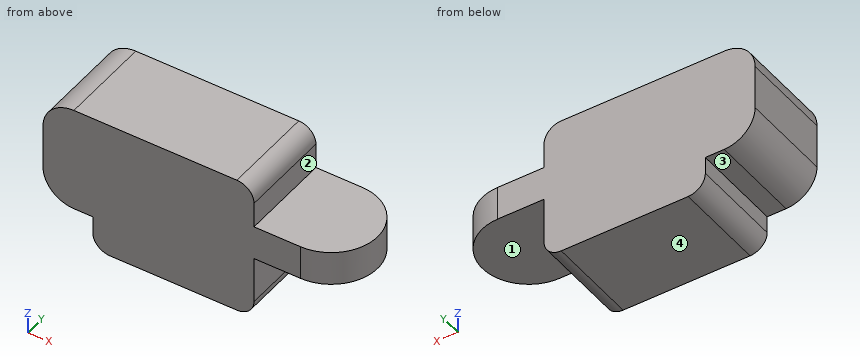
```python
from build123d import *

# Parameters (mm, degrees)
BOSS_EXTRUDE1_DEPTH      = 34.29
BOSS_EXTRUDE1_DEPTH_BACK = 34.29
CUT_EXTRUDE1_DEPTH       = 203.631037198
CUT_EXTRUDE1_DEPTH_BACK  = 203.631037198


with BuildPart() as part:
    # Sketch1 → Boss-Extrude1 (new, two sides: drawn at the far end of the back side and taken through both)
    with BuildSketch(Plane(origin=(0, 0, 0), x_dir=(1, 0, 0), z_dir=(0, 1, 0)).offset(-BOSS_EXTRUDE1_DEPTH_BACK)):
        with BuildLine():
            Line((-34.29, -12.7), (34.29, -12.7))
            Line((34.29, -12.7), (34.29, 12.7))
            Line((34.29, 12.7), (-34.29, 12.7))
            Line((-34.29, 12.7), (-34.29, 47.244))
            ThreePointArc((-34.29, 47.244), (-38.009743879, 56.224256121), (-46.99, 59.944))
            Line((-46.99, 59.944), (-140.97, 59.944))
            ThreePointArc((-140.97, 59.944), (-149.950256121, 56.224256121), (-153.67, 47.244))
            Line((-153.67, 47.244), (-153.67, 34.544))
            Line((-153.67, 34.544), (-167.64, 34.544))
            ThreePointArc((-167.64, 34.544), (-183.804461018, 27.848461018), (-190.5, 11.684))
            Line((-190.5, 11.684), (-190.5, -21.336))
            ThreePointArc((-190.5, -21.336), (-183.804461018, -37.500461018), (-167.64, -44.196))
            Line((-167.64, -44.196), (-46.99, -44.196))
            ThreePointArc((-46.99, -44.196), (-38.009743879, -40.476256121), (-34.29, -31.496))
            Line((-34.29, -31.496), (-34.29, -12.7))
        make_face()
    extrude(amount=BOSS_EXTRUDE1_DEPTH + BOSS_EXTRUDE1_DEPTH_BACK)

    # Sketch2 → Cut-Extrude1 (cut, two sides: drawn at the far end of the back side and taken through both)
    with BuildSketch(Plane.XY.offset(-CUT_EXTRUDE1_DEPTH_BACK)):
        with BuildLine():
            Line((0, 34.29), (44.29, 34.29))
            Line((44.29, 34.29), (44.29, -34.29))
            Line((44.29, -34.29), (0, -34.29))
            ThreePointArc((0, -34.29), (34.29, 0), (0, 34.29))
        make_face()
    extrude(amount=CUT_EXTRUDE1_DEPTH + CUT_EXTRUDE1_DEPTH_BACK, mode=Mode.SUBTRACT)


solid = part.part
```
Could you check a few things on this model? Use its own coordinates, in mm. Face numbers are marked on the shaded views. A direction names the side the tool comes from. Round coordinates to 2 decimals unless told otherwise and drop trailing zeros. Loops run counter-clockwise (first coordinate to the right, second up) from the corner with the lowest first, then second, coordinate; pieces in that order, holes last. Notation, with made-up numbers: M -35.75,23 L 13.25,23 A16 ccw 13.25,39 Z; hole C 45.5,-23 d4. An arc over 180 degrees is marked long. Put each result on its own line as item: value.
Q1. For pin 1 (5 mm diameter, centred on x = -2, y = -16.5, fed in from +Z); pin 2 (10 mm diameter, centred on y = -14, z = -42.5, fed in from -X); pin 3 (17.5 mm diameter, centred on y = -9.5, z = -32.5, fed in from +X), each with a flat end and sliding along its axis, tell me the tip position at first contact or that it passes through.
Check result:
pin 1: z = 12.7
pin 2: x = -153.67
pin 3: x = -34.29
Q2. Imagine slicing it at A-A (y = 0). Write out the boundary of the cut face in (x, z).
Check result:
outline: M -190.5,-11.68 A22.86 ccw -167.64,-34.54 L -153.67,-34.54 L -153.67,-47.24 A12.7 ccw -140.97,-59.94 L -46.99,-59.94 A12.7 ccw -34.29,-47.24 L -34.29,-12.7 L 34.29,-12.7 L 34.29,12.7 L -34.29,12.7 L -34.29,31.5 A12.7 ccw -46.99,44.2 L -167.64,44.2 A22.86 ccw -190.5,21.34 Z
Q3. On a 3-axis mill with a long thin cutter (end or side, diameter ignored), from which of +Z, -Z, +X, -X, +Y, -Y can I reach the whole of each face in a straight line? I mean the marked faces 1, 2, 3 and 4. Say none if no direction works.
Check result:
face 1: -Z, +X, +Y, -Y
face 2: +Z, +X, +Y, -Y
face 3: -Z, -X, +Y, -Y
face 4: -Z, +X, -X, +Y, -Y
Q4. Imagine slicing it at B-B (y = 13). Write out the boundary of the cut face in (x, z), then the cut area to 3 significant figures.
Check result:
outline: M -190.5,-11.68 A22.86 ccw -167.64,-34.54 L -153.67,-34.54 L -153.67,-47.24 A12.7 ccw -140.97,-59.94 L -46.99,-59.94 A12.7 ccw -34.29,-47.24 L -34.29,-12.7 L 31.73,-12.7 L 31.73,12.7 L -34.29,12.7 L -34.29,31.5 A12.7 ccw -46.99,44.2 L -167.64,44.2 A22.86 ccw -190.5,21.34 Z
area: 16,700 mm2
Q5. I need wall thicknesses on probe 1 along Z at (x, y) = (-10, -24.5); probe 2 along X at (y, z) = (-9.5, 14); probe 3 along X at (y, z) = (21, -42). Which ranges of each line are inside material? Lowest first, please.
Check result:
probe 1: -12.7 to 12.7
probe 2: -190.5 to -34.29
probe 3: -153.67 to -34.29
Q6. Imagine slicing it at C-C (z = -26.5). Write out the boundary of the cut face in (x, y).
Check result:
outline: M -185.05,-34.29 L -34.29,-34.29 L -34.29,34.29 L -185.05,34.29 Z
